Autodesk Inventor part; units mm, degrees
ref_plane "YZ Plane" through (0, 0, 0) normal (1, 0, 0) x (0, 1, 0)
ref_plane "XZ Plane" through (0, 0, 0) normal (0, 1, 0) x (-1, 0, 0)
ref_plane "XY Plane" through (0, 0, 0) normal (0, 0, 1) x (1, 0, 0)
sketch "Szkic1" plane through (0, 0, 0) normal (0, 0, 1) x (1, 0, 0)
  line L0 (0, 0) -> (64, 0) construction
  line L1 (64, 0) -> (64, 70) construction
  line L2 (64, 70) -> (0, 70) construction
  line L3 (0, 70) -> (0, 0) construction
  line L4 (0, 0) -> (6, 0) construction
  line L5 (6, 70) -> (0, 70) construction
  line L6 (0, 70) -> (0, 0) construction
  line L7 (6, 0) -> (174, 0) construction
  line L8 (0, 0) -> (64, 0) construction
  line L9 (64, 0) -> (64, 6) construction
  line L10 (64, 6) -> (0, 6) construction
  line L11 (0, 6) -> (0, 0) construction
  line L12 (0, 6) -> (168, 6) construction
  line L13 (168, 6) -> (168, 174) construction
  line L14 (168, 174) -> (0, 174) construction
  line L15 (0, 174) -> (0, 6) construction
  line L16 (84, 174) -> (84, 6) construction
  circle A0 centre (84, 90) radius 65 construction
  line L17 (0, 0) -> (64, 0)
  line L18 (64, 0) -> (64, 28.1534)
  line L19 (0, 0) -> (0, 70)
  line L20 (0, 70) -> (22.1534, 70)
  arc A1 (22.1534, 70) -> (64, 28.1534) centre (84, 90) ccw
  dimension "d13" = 64
  dimension "d14" = 70
  dimension "d19" = 6
  dimension "d20" = 168
  dimension "d21" = 168
  dimension "d22" = 130
extrude "Wyciągnięcie proste1" add sketch "Szkic1" along normal blind 6
properties part number "Naroznik_60x54"
Could you check a few things on this model? Use its own coordinates, in mm. Coordinates: 2 decimals unless noted, no trailing zeros. Loops run counter-clockwise (first coordinate to the right, second up) from the corner with the lowest first, then second, coordinate; pieces in that order, holes last.
1. Imagine slicing it at A-A (z = 3.2). Please give me the cut outline in (x, y).
2. I need wall thicknesses on L1, parallel to X at y = 34, z = 4.5; L2, parallel to Y at x = 33.5, z = 2.9; L3, parallel to Y at x = 46, z = 5.6. Which ranges of each line are inside material? Lowest first, please.
3. Imagine slicing it at B-B (x = 34.5). Please give me the cut outline in (y, z), and give its area (3 significant figures).
4. Imagine slicing it at C-C (y = 44). Please give me the cut outline in (x, z).
5. For P1, Ø4, axis at x = 32.5, y = 26, coming from the -Z side; P2, Ø2, axis at y = 50, z = 1.5, coming from the +X side, each with a flat end and sliding along its axis, tell me the tip position at first contact or that it passes through.
Computed values:
1. outline: (0, 0) - (64, 0) - (64, 28.15) arc R65 cw to (22.15, 70) - (0, 70) - close
2. L1: x = 0 to 51
2. L2: y = 0 to 49.08
2. L3: y = 0 to 37.26
3. outline: (0, 0) - (47.87, 0) - (47.87, 6) - (0, 6) - close
3. area: 287 mm2
4. outline: (0, 0) - (38.08, 0) - (38.08, 6) - (0, 6) - close
5. P1: stops at z = 0
5. P2: stops at x = 33.56
